The listing builds one solid part. Answer for the finished solid, in the listing's coordinates (mm). A direction names the side the tool comes from. Round coordinates to 2 decimals unless told otherwise and drop trailing zeros. Write each loop counter-clockwise with the first axis right and the second up, starting at its lowest first coordinate (ties: lowest second). Pieces come first, ordered by that corner, then holes.
(1) A cutting plane is placed at A-A, the plane x = 127.5. Give the vertices of the cut face in (y, z), and give its area (3 significant figures).
(2) The mould has two halves that part along Y. Classify faces 5 (the face through (120.182, 186.854, 1.479)), 6 (the face through (108, 181.089, 1)), 7 (the face through (110.375, 206, 1)): +Y half, -Y half, draft (parallel to the pull), parting line (faces both ways), or undercut.
(3) Each of these flat-tipped pins is pushed along its axis until it touches: pin 1 Ø2.5 at (x, y) = (128.38, 200.59) entering from +Z; pin 2 Ø1.5 at (x, z) = (140.5, 2) entering from -Y; pin 3 Ø0.9 at (x, z) = (109.5, 2) entering from +Y; pin 4 Ø0.9 at (y, z) = (204.5, 1) entering from +X. Where does it stop, or does it pass through?
(4) For faces 1 (the face through (140, 181.089, 1)), 2 (the face through (110.375, 180, 1)), 3 (the face through (140.375, 204, 1)), 4 (the face through (114.875, 201, 1)), determine the directions among +Z, -Z, +X, -X, +Y, -Y from which every point of the face is accessible in a straight line to the end or side of a thin tool.
(5) A cutting plane is placed at B-B, the plane z = 1.7. Give the number of separate pieces and of enclosed holes in the cut face, and give its area (3 significant figures).
(6) Find the intervals of material crossed by probe 1 along Y at (x, z) = (128, 2.6); probe 2 along X at (y, z) = (201, 0.15); probe 3 along Y at (x, z) = (129, 2.4), in increasing order.
from build123d import *

# Parameters (mm, degrees)
MODEL_R                 = 1.5
SALIENTE_EXTRUIR1_DEPTH = 3


with BuildPart() as part:
    # Model → Saliente-Extruir1 (new body)
    with BuildSketch(Plane.XY):
        with BuildLine():
            ThreePointArc((110.375172306, 199.089330986), (107.193819506, 197.771939094), (105.875172656, 194.59110626))
            Line((105.875172656, 194.59110626), (105.875172656, 181.089330986))
            Line((105.875172656, 181.089330986), (110.375172306, 181.089330986))
            Line((110.375172306, 181.089330986), (110.375172306, 179.589330986))
            Line((110.375172306, 179.589330986), (137.375172656, 179.589330986))
            Line((137.375172656, 179.589330986), (137.375172656, 181.089330986))
            Line((137.375172656, 181.089330986), (141.875172656, 181.089330986))
            Line((141.875172656, 181.089330986), (141.875172656, 194.589330986))
            ThreePointArc((141.875172656, 194.589330986), (140.554536568, 197.773926028), (137.367774797, 199.089325081))
            Line((137.367774797, 199.089325081), (133.625176703, 199.089319857))
            ThreePointArc((133.625176703, 199.089319857), (133.09484632, 199.308989056), (132.875175691, 199.839318846))
            Line((132.875175691, 199.839318846), (132.875173667, 201.339318846))
            ThreePointArc((132.875173667, 201.339318846), (133.094842866, 201.869649228), (133.625172656, 202.089319857))
            Line((133.625172656, 202.089319857), (137.375178726, 202.089324916))
            ThreePointArc((137.375178726, 202.089324916), (138.980875531, 202.385553219), (140.375172656, 203.23522902))
            Line((140.375172656, 203.23522902), (140.375172656, 205.089330986))
            Line((140.375172656, 205.089330986), (137.375172656, 205.089330986))
            Line((137.375172656, 205.089330986), (137.375165869, 206.589324916))
            Line((137.375165869, 206.589324916), (110.375172306, 206.589330986))
            Line((110.375172306, 206.589330986), (110.375172306, 205.089330986))
            Line((110.375172306, 205.089330986), (107.375172306, 205.089330986))
            Line((107.375172306, 205.089330986), (107.375172306, 203.23522902))
            ThreePointArc((107.375172306, 203.23522902), (108.769472902, 202.385555371), (110.375172306, 202.089330986))
            Line((110.375172306, 202.089330986), (114.125172656, 202.089330986))
            ThreePointArc((114.125172656, 202.089330986), (114.655502742, 201.869661072), (114.875172656, 201.339330986))
            Line((114.875172656, 201.339330986), (114.875172656, 199.839330986))
            ThreePointArc((114.875172656, 199.839330986), (114.655502742, 199.3090009), (114.125172656, 199.089330986))
            Line((114.125172656, 199.089330986), (110.375172306, 199.089330986))
        make_face()
        with Locations((110.375172306, 185.589330986)):
            Circle(MODEL_R, mode=Mode.SUBTRACT)
        with Locations((119.375172306, 185.589330986)):
            Circle(MODEL_R, mode=Mode.SUBTRACT)
        with Locations((128.375172306, 185.589330986)):
            Circle(MODEL_R, mode=Mode.SUBTRACT)
        with Locations((137.375172306, 185.589330986)):
            Circle(MODEL_R, mode=Mode.SUBTRACT)
        with Locations((110.375172306, 194.589330986)):
            Circle(MODEL_R, mode=Mode.SUBTRACT)
        with Locations((119.375172306, 194.589330986)):
            Circle(MODEL_R, mode=Mode.SUBTRACT)
        with Locations((119.375172656, 200.589330986)):
            Circle(MODEL_R, mode=Mode.SUBTRACT)
        with Locations((128.375172306, 194.589330986)):
            Circle(MODEL_R, mode=Mode.SUBTRACT)
        with Locations((137.375172481, 194.589330986)):
            Circle(MODEL_R, mode=Mode.SUBTRACT)
        with Locations((128.375172656, 200.589330986)):
            Circle(MODEL_R, mode=Mode.SUBTRACT)
    extrude(amount=SALIENTE_EXTRUIR1_DEPTH)


solid = part.part
Solutions:
1. outline: (179.59, 0) - (184.37, 0) - (184.37, 3) - (179.59, 3) - close; (186.81, 0) - (193.37, 0) - (193.37, 3) - (186.81, 3) - close; (195.81, 0) - (199.37, 0) - (199.37, 3) - (195.81, 3) - close; (201.81, 0) - (206.59, 0) - (206.59, 3) - (201.81, 3) - close
1. area: 59.1 mm2
2. face 5: undercut
2. face 6: -Y half
2. face 7: draft
3. pin 1: passes through
3. pin 2: stops at y = 181.09
3. pin 3: stops at y = 205.09
3. pin 4: stops at x = 140.38
4. face 1: +Z, -Z, +X, -Y
4. face 2: +Z, -Z, -X, -Y
4. face 3: +Z, -Z, +X, +Y
4. face 4: +Z, -Z, -X
5. separate pieces: 1
5. enclosed holes: 10
5. area: 801 mm2
6. probe 1: y = 179.59 to 184.14, 187.04 to 193.14, 196.04 to 199.14, 202.04 to 206.59
6. probe 2: x = 114.88 to 117.93, 120.82 to 126.93, 129.82 to 132.88
6. probe 3: y = 179.59 to 184.23, 186.95 to 193.23, 195.95 to 199.23, 201.95 to 206.59
